Part model, mm, in its own coordinate system. Face numbers are marked on the shaded views. A direction names the side the tool comes from. Give positions to 0.01 mm unless a question says otherwise; leave off trailing zeros. Order: outer loops, then holes, each group sorted by start corner. A loop starts at its lowest first (then second) coordinate and runs counter-clockwise, first axis right, second up.
1. Slice it at C-C on z = 5.5. Give the number of separate pieces and of enclosed holes in the cut face, and give its area (3 significant figures).
2. Mould opens along X. For the marked faces 1, 2 and 3 say: +X half, -X half, draft (parallel to the pull), parting line (faces both ways), or undercut.
3. Which spindle directions (+Z, -Z, +X, -X, +Y, -Y) get a long thin tool onto all of the face, cutting with end or side? Do the marked faces 4 and 5. Say none if no direction does.
4. Slice it at A-A on x = 6.5. List the corners of the cut face in (y, z), and give its area (3 significant figures).
5. Drop flat-ended pins along their axis: pin 1 Ø3 at (x, z) = (-12, -18) entering from +Y; pin 2 Ø6 at (y, z) = (1, -0.5) entering from -X; pin 3 Ø6 at (x, z) = (-14.5, -23.5) entering from +Y; pin 4 Ø1.6 at (x, y) = (1.5, 2) entering from -Z. Give the stop position or say it passes through.
6. Probe line 1 (X direction, y = -0.5, z = 5); line 2 (X direction, y = 4.75, z = 5); line 3 (Y direction, x = -16.5, z = 1.5). List the from-to ranges inside material, lowest first.
7. Slice it at B-B on x = -12. List the corners of the cut face in (y, z), and give its area (3 significant figures).
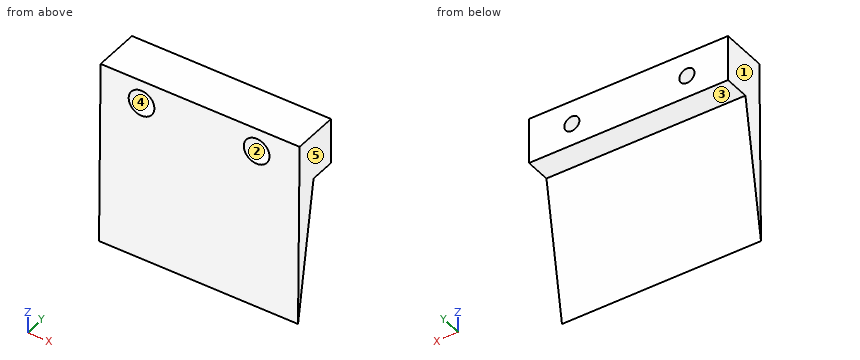
from build123d import *

# Parameters (mm, degrees)
BOSS_EXTRUDE1_DEPTH                            = 21.5
SKETCH4_R                                      = 0.685
CUT_EXTRUDE1_DEPTH                             = 11.401915701
CBORE_FOR_4_SOCKET_HEAD_CAP_SCREW1_D           = 3.2639
CBORE_FOR_4_SOCKET_HEAD_CAP_SCREW1_CBORE_D     = 5.55752
CBORE_FOR_4_SOCKET_HEAD_CAP_SCREW1_CBORE_DEPTH = 6.844792


with BuildPart() as part:
    # Sketch2 → Boss-Extrude1 (new body, symmetric)
    with BuildSketch(Plane(origin=(0, 0, 0), x_dir=(0, 0, -1), z_dir=(1, 0, 0))):
        Polygon((0, 0), (29.596811018, -4.901915701), (-9.9, -4.4), (-9.9, 5.5), (0, 5.5), align=None)
    extrude(amount=BOSS_EXTRUDE1_DEPTH, both=True)

    # Sketch4 → Cut-Extrude1 (cut, through all)
    with BuildSketch(Plane(origin=(0, 5.5, 0), x_dir=(1, 0, 0), z_dir=(0, 1, 0))):
        with Locations((-12.615, -4.95)):
            Circle(SKETCH4_R)
        with Locations((12.255, -4.95)):
            Circle(SKETCH4_R)
    extrude(amount=-CUT_EXTRUDE1_DEPTH, mode=Mode.SUBTRACT)

    # CBORE for #4 Socket Head Cap Screw1 (through all)
    with Locations(Plane(origin=(0, -4.525076009, 0.057503546), x_dir=(-1, 0, 0), z_dir=(0, -0.999919266, 0.012706727))):
        with Locations((12.615, -4.892891475), (-12.255, -4.892891475)):
            CounterBoreHole(CBORE_FOR_4_SOCKET_HEAD_CAP_SCREW1_D / 2, CBORE_FOR_4_SOCKET_HEAD_CAP_SCREW1_CBORE_D / 2, CBORE_FOR_4_SOCKET_HEAD_CAP_SCREW1_CBORE_DEPTH)


solid = part.part
Data:
1. separate pieces: 3
1. enclosed holes: 0
1. area: 335 mm2
2. face 1: -X half
2. face 2: undercut
2. face 3: draft
3. face 4: none
3. face 5: +Z, -Z, +X, +Y, -Y
4. outline: (-4.9, -29.6) - (0, 0) - (5.5, 0) - (5.5, 9.9) - (-4.4, 9.9) - close
4. area: 166 mm2
5. pin 1: stops at y = -2.73
5. pin 2: stops at x = -21.5
5. pin 3: stops at y = -3.4
5. pin 4: stops at z = 0
6. line 1: x = -21.5 to -15.39, -9.84 to 9.48, 15.03 to 21.5
6. line 2: x = -21.5 to -14.24, -10.99 to 10.63, 13.88 to 21.5
6. line 3: y = -4.51 to 5.5
7. outline: (-4.9, -29.6) - (0, 0) - (5.5, 0) - (5.5, 3.31) - (2.36, 3.35) - (2.35, 2.15) - (-4.5, 2.24) - close; (-4.43, 7.66) - (2.42, 7.57) - (2.4, 6.37) - (5.5, 6.34) - (5.5, 9.9) - (-4.4, 9.9) - close
7. area: 119 mm2
